Source: CAD feature listing. Evaluate the final solid. Frame: model axes, mm. Face numbers are marked on the shaded views. A direction names the side the tool comes from. Give positions to 0.01 mm unless a question says otherwise; leave off trailing zeros. Order: outer loops, then holes, each group sorted by start corner. A loop starts at its lowest first (then second) coordinate and runs counter-clockwise, first axis right, second up. Notation, with made-up numbers: (75, -13.75) - (93, -13.75) arc R13 cw to (93, -7.75) - close; hole circle Ø2 at (73, -37). An arc over 180 degrees is marked (long way). Write each question's results on one line, items separated by ' | '. Start each with the question number.
Item 1: Set-up query: the marked faces 1 and 2. Return all of +Z, -Z, +X, -X, +Y, -Y with unobstructed straight access to the full face (end or side cutting, diameter ignored); none if empty.
Item 2: Line query: line 1 along Y through (x, z) = (11, 0.5); line 2 along Z through (x, y) = (-62.5, 32) (3 decimals); line 3 along X through (y, z) = (30, 0.4). Output: solid intervals per line, ascending.
Item 3: Section B-B on y = -26. Output: boundary loops of the cut face in (x, z) (1 decimal).
Item 4: Section A-A on x = -12. Output: boundary loops of the cut face in (y, z) (1 decimal), and give its area (3 significant figures).
Item 5: Contact query for flat-ended pins moving along their axis: pin 1 Ø2.5 at (x, y) = (15.88, 68.72) entering from -Z; pin 2 Ø5 at (x, y) = (-4.76, -35.26) entering from +Z. Output: stop coordinate, or through.
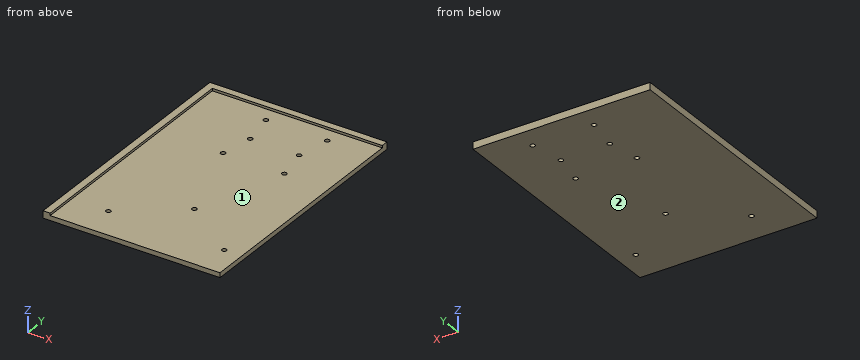
```python
from build123d import *

# Parameters (mm, degrees)
F0_W     = 114.3
F0_H     = 165.1
F0_R     = 1.5875
F1_DEPTH = 3.175
F2_DEPTH = 1.5875


with BuildPart() as f1:
    # F0 (on Top) → F1 (new body)
    with BuildSketch(Plane.XY):
        with Locations((-11.107412, -3.511809)):
            Rectangle(F0_W, F0_H)
        with Locations((-43.670212, -63.836809)):
            Circle(F0_R, mode=Mode.SUBTRACT)
        with Locations((34.155388, -63.836809)):
            Circle(F0_R, mode=Mode.SUBTRACT)
        with Locations((-4.757412, -35.261809)):
            Circle(F0_R, mode=Mode.SUBTRACT)
        with Locations((-25.394912, 25.060651)):
            Circle(F0_R, mode=Mode.SUBTRACT)
        with Locations((-21.250462, 46.493171)):
            Circle(F0_R, mode=Mode.SUBTRACT)
        with Locations((-25.394912, 68.718171)):
            Circle(F0_R, mode=Mode.SUBTRACT)
        with Locations((15.880088, 25.060651)):
            Circle(F0_R, mode=Mode.SUBTRACT)
        with Locations((11.585386, 46.493171)):
            Circle(F0_R, mode=Mode.SUBTRACT)
        with Locations((15.880088, 68.718171)):
            Circle(F0_R, mode=Mode.SUBTRACT)
        Polygon((-68.257412, -86.061809), (-68.257412, 79.038191), (46.042588, 79.038191), (46.042588, 83.813391), (-73.019912, 83.813391), (-73.019912, -86.061809), align=None)
    extrude(amount=-F1_DEPTH)

    # F0 (on Top) → F2 (join)
    with BuildSketch(Plane.XY):
        Polygon((-68.257412, -86.061809), (-68.257412, 79.038191), (46.042588, 79.038191), (46.042588, 83.813391), (-73.019912, 83.813391), (-73.019912, -86.061809), align=None)
    extrude(amount=F2_DEPTH)


solid = f1.part
```
Evaluation:
1) face 1: +Z, +X, -Y | face 2: -Z, +X, -X, +Y, -Y
2) line 1: y = 79.04 to 83.81 | line 2: z = -3.175 to 0 | line 3: x = -73.02 to -68.26
3) outline: (-73, -3.2) - (46, -3.2) - (46, 0) - (-68.3, 0) - (-68.3, 1.6) - (-73, 1.6) - close
4) outline: (-86.1, -3.2) - (83.8, -3.2) - (83.8, 1.6) - (79, 1.6) - (79, 0) - (-86.1, 0) - close | area: 547 mm^2
5) pin 1: passes through | pin 2: stops at z = 0
